Could you check a few things on this model? Use its own coordinates, in mm. Face numbers are marked on the shaded views. A direction names the side the tool comes from. Round coordinates to 2 decimals unless told otherwise and drop trailing zeros. Loops run counter-clockwise (first coordinate to the right, second up) from the corner with the lowest first, then second, coordinate; pieces in that order, holes last. Notation, with made-up numbers: M 71.25,62.5 L 100.25,62.5 A21 ccw 100.25,84.5 Z; hole C 59,44.5 d8. An arc over 180 degrees is marked long. Return JSON: item names as keys, results as strings. Group by question number.
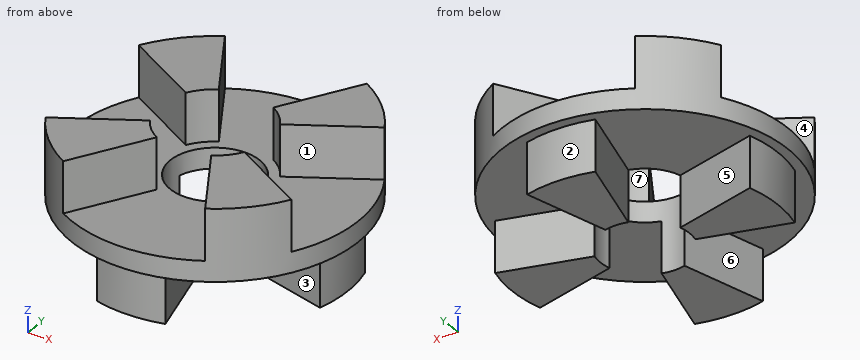
```python
from build123d import *

# Parameters (mm, degrees)
F3_DEPTH = 127
F5_DEPTH = 127


with BuildPart() as f1:
    # F0 (on Front) → F1 (revolve)
    with BuildSketch(Plane.XZ):
        Polygon((136.525, 177.8), (111.125, 177.8), (111.125, 0), (330.2, 0), (330.2, 127), (355.6, 127), (355.6, 304.8), (136.525, 304.8), align=None)
    revolve(axis=Axis((0, 0, 359.9156904304), (0, 0, 1)))

    # F2 (on face) → F3 (cut)
    with BuildSketch(Plane.XY.offset(304.8)):
        with BuildLine():
            ThreePointArc((-307.9586335857, 177.8), (-355.6, 0), (-307.9586335857, -177.8))
            Line((-307.9586335857, -177.8), (-118.2341182517, -68.2625))
            ThreePointArc((-118.2341182517, -68.2625), (-136.525, 0), (-118.2341182517, 68.2625))
            Line((-118.2341182517, 68.2625), (-307.9586335857, 177.8))
        make_face()
        with BuildLine():
            Line((-68.2625, -118.2341182517), (-177.8, -307.9586335857))
            ThreePointArc((-177.8, -307.9586335857), (0, -355.6), (177.8, -307.9586335857))
            Line((177.8, -307.9586335857), (68.2625, -118.2341182517))
            ThreePointArc((68.2625, -118.2341182517), (0, -136.525), (-68.2625, -118.2341182517))
        make_face()
        with BuildLine():
            ThreePointArc((177.8, 307.9586335857), (0, 355.6), (-177.8, 307.9586335857))
            Line((-177.8, 307.9586335857), (-68.2625, 118.2341182517))
            ThreePointArc((-68.2625, 118.2341182517), (0, 136.525), (68.2625, 118.2341182517))
            Line((68.2625, 118.2341182517), (177.8, 307.9586335857))
        make_face()
        with BuildLine():
            Line((307.9586335857, 177.8), (118.2341182517, 68.2625))
            ThreePointArc((118.2341182517, 68.2625), (131.8730234341, 35.3352701326), (136.525, 0))
            ThreePointArc((136.525, 0), (131.8730234341, -35.3352701326), (118.2341182517, -68.2625))
            Line((118.2341182517, -68.2625), (307.9586335857, -177.8))
            ThreePointArc((307.9586335857, -177.8), (343.4832238284, -92.0360524385), (355.6, 0))
            ThreePointArc((355.6, 0), (343.4832238284, 92.0360524385), (307.9586335857, 177.8))
        make_face()
        with BuildLine():
            ThreePointArc((355.6, 0), (343.4832238284, -92.0360524385), (307.9586335857, -177.8))
            Line((307.9586335857, -177.8), (329.9556788419, -190.5))
            ThreePointArc((329.9556788419, -190.5), (381, 0), (329.9556788419, 190.5))
            Line((329.9556788419, 190.5), (307.9586335857, 177.8))
            ThreePointArc((307.9586335857, 177.8), (343.4832238284, 92.0360524385), (355.6, 0))
        make_face()
    extrude(amount=-F3_DEPTH, mode=Mode.SUBTRACT)

    # F4 (on face) → F5 (cut)
    with BuildSketch(Plane(origin=(0, 0, 0), x_dir=(1, 0, 0), z_dir=(0, 0, -1))):
        with BuildLine():
            Line((-28.761266387, 107.3385074464), (-85.4620486929, 318.9487078407))
            ThreePointArc((-85.4620486928, 318.9487078407), (-233.4866591478, 233.4866591478), (-318.9487078407, 85.4620486929))
            Line((-318.9487078407, 85.4620486929), (-107.3385074464, 28.761266387))
            ThreePointArc((-107.3385074464, 28.761266387), (-78.5772410594, 78.5772410594), (-28.761266387, 107.3385074464))
        make_face()
        with BuildLine():
            Line((107.3385074464, 28.761266387), (318.9487078407, 85.4620486929))
            ThreePointArc((318.9487078406, 85.4620486929), (233.4866591478, 233.4866591478), (85.4620486928, 318.9487078407))
            Line((85.4620486929, 318.9487078407), (28.761266387, 107.3385074464))
            ThreePointArc((28.761266387, 107.3385074464), (78.5772410594, 78.5772410594), (107.3385074464, 28.761266387))
        make_face()
        with BuildLine():
            ThreePointArc((85.4620486928, -318.9487078407), (233.4866591478, -233.4866591478), (318.9487078406, -85.4620486929))
            Line((318.9487078407, -85.4620486929), (107.3385074464, -28.761266387))
            ThreePointArc((107.3385074464, -28.761266387), (78.5772410594, -78.5772410594), (28.761266387, -107.3385074464))
            Line((28.761266387, -107.3385074464), (85.4620486929, -318.9487078407))
        make_face()
        with BuildLine():
            ThreePointArc((-318.9487078407, -85.4620486929), (-233.4866591478, -233.4866591478), (-85.4620486928, -318.9487078407))
            Line((-85.4620486929, -318.9487078407), (-28.761266387, -107.3385074464))
            ThreePointArc((-28.761266387, -107.3385074464), (-78.5772410594, -78.5772410594), (-107.3385074464, -28.761266387))
            Line((-107.3385074464, -28.761266387), (-318.9487078407, -85.4620486929))
        make_face()
    extrude(amount=-F5_DEPTH, mode=Mode.SUBTRACT)


solid = f1.part
```
1. If we section it at A-A, the plane y = 0: Please give me the cut outline in (x, z) (3 decimals).
2. I need wall thicknesses on probe 1 along X at (y, z) = (0, 66.5) (3 decimals); probe 2 along Z at (x, y) = (123.5, 32); probe 3 along X at (y, z) = (-149.5, 256.5). Which ranges of each line are inside material? Lowest first, please.
3. On a 3-axis mill with a long thin cutter (end or side, diameter ignored), from which of +Z, -Z, +X, -X, +Y, -Y can I reach the whole of each face in a straight line? I mean the marked faces 5, 6 and 7. Say none if no direction works.
4. We'd pull the mould along Y, two halves only. Please class the marked faces 1, 2, 3 and 4: +Y half, -Y half, draft (parallel to the pull), parting line (faces both ways), or undercut.
5. If we section it at C-C, the plane z = 220: Give the number of separate pieces and of enclosed holes in the cut face, then the cut area to 3 significant figures.
6. I'm going to push flat-ended pins straight in: pin 1 Ø5 at (y, z) = (77.5, 129.5) entering from +X; pin 2 Ø2 at (x, z) = (253, 191.5) entering from -Y; pin 3 Ø12 at (y, z) = (-106, 178.5) entering from +X. Where does each tip first touch, or does it pass through?
Geometry results:
{
 "1": {"outline": "M -355.6,127 L -330.2,127 L -330.2,0 L -111.125,0 L -111.125,177.8 L -355.6,177.8 Z; M 111.125,0 L 330.2,0 L 330.2,127 L 355.6,127 L 355.6,177.8 L 111.125,177.8 Z"},
 "2": {"probe 1": "-330.2 to -111.125, 111.125 to 330.2", "probe 2": "0 to 177.8", "probe 3": "-258.94 to -86.31, 86.31 to 258.94"},
 "3": {"face 5": "-Z, +Y", "face 6": "-Z, -X", "face 7": "+Z"},
 "4": {"face 1": "undercut", "face 2": "+Y half", "face 3": "-Y half", "face 4": "undercut"},
 "5": {"separate pieces": "4", "enclosed holes": "0", "area": "113,000 mm^2"},
 "6": {"pin 1": "x = 347.6", "pin 2": "y = -250.89", "pin 3": "x = 341.24"}
}
